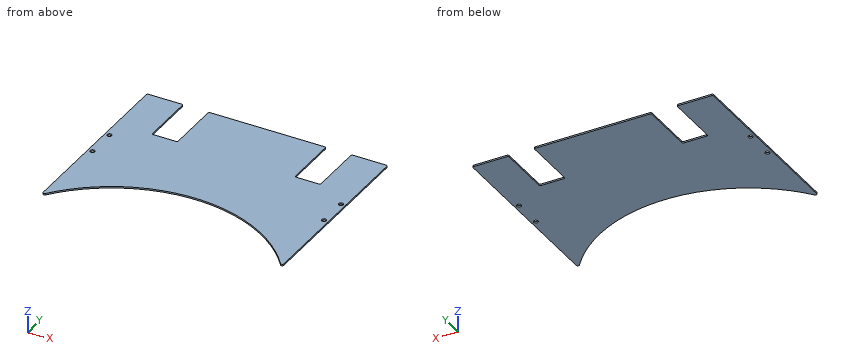
from build123d import *

# Parameters (mm, degrees)
SKETCH_1_W           = 160
SKETCH_1_H           = 104
EXTRUDE_1_DEPTH      = 0.5
SKETCH_12_R          = 99.362749495
CUT_EXTRUDE_6_DEPTH  = 1
EXTRUDE_3_DEPTH      = 1
SKETCH_17_W          = 17
SKETCH_17_H          = 92.283863988
CUT_EXTRUDE_9_DEPTH  = 1
SKETCH_21_R          = 1.525
CUT_EXTRUDE_14_DEPTH = 10
FILLET_4_R           = 1


with BuildPart() as part:
    # 草图1 → 凸台-拉伸1 (new, symmetric)
    with BuildSketch(Plane.XY):
        Rectangle(SKETCH_1_W, SKETCH_1_H)
    extrude(amount=EXTRUDE_1_DEPTH, both=True)

    # 草图12 → 切除-拉伸6 (cut)
    with BuildSketch(Plane(origin=(0, 0, -0.5), x_dir=(-1, 0, 0), z_dir=(0, 0, -1))):
        with Locations((0, -133)):
            Circle(SKETCH_12_R)
    extrude(amount=-CUT_EXTRUDE_6_DEPTH, mode=Mode.SUBTRACT)

    # 草图13 → 凸台-拉伸3 (add)
    with BuildSketch(Plane(origin=(0, 0, -0.5), x_dir=(-1, 0, 0), z_dir=(0, 0, -1))):
        with BuildLine():
            Line((80, -52), (80, -74.068209027))
            ThreePointArc((80, -74.068209027), (69.654320002, -62.139350184), (57.549595892, -52))
            Line((57.549595892, -52), (80, -52))
        make_face()
    extrude_3 = extrude(amount=-EXTRUDE_3_DEPTH)

    # 镜向2: 凸台-拉伸3 across plane
    add(extrude_3.mirror(Plane(origin=(0, 0, 0), x_dir=(0, 0, 1), z_dir=(1, 0, 0))))

    # 草图17 → 切除-拉伸9 (cut)
    with BuildSketch(Plane(origin=(0, 0, -0.5), x_dir=(-1, 0, 0), z_dir=(0, 0, -1))):
        with Locations((-47.5, 61.084572681)):
            Rectangle(SKETCH_17_W, SKETCH_17_H)
    cut_extrude_9 = extrude(amount=-CUT_EXTRUDE_9_DEPTH, mode=Mode.SUBTRACT)

    # 镜向4: 切除-拉伸9 across plane
    add(cut_extrude_9.mirror(Plane(origin=(0, 0, 0), x_dir=(0, 0, 1), z_dir=(1, 0, 0))), mode=Mode.SUBTRACT)

    # 草图21 → 切除-拉伸14 (cut)
    with BuildSketch(Plane(origin=(0, 0, -0.5), x_dir=(-1, 0, 0), z_dir=(0, 0, -1))):
        with Locations((-77, 2)):
            Circle(SKETCH_21_R)
        with Locations((-77, -18)):
            Circle(SKETCH_21_R)
        with Locations((77, -18)):
            Circle(SKETCH_21_R)
        with Locations((77, 2)):
            Circle(SKETCH_21_R)
    extrude(amount=-CUT_EXTRUDE_14_DEPTH, mode=Mode.SUBTRACT)

    # 圆角4
    fillet_4_edges = [part.edges().sort_by_distance(p)[0] for p in [
        (-80, -74.068209027, 0),
        (80, -74.068209027, 0),
        (39, 52, 0),
        (56, 52, 0),
        (56, 14.942640687, 0),
        (39, 14.942640687, 0),
        (-39, 14.942640687, 0),
        (-56, 14.942640687, 0),
        (-56, 52, 0),
        (-39, 52, 0),
        (-80, 52, 0),
        (80, 52, 0),
    ]]
    fillet(fillet_4_edges, radius=FILLET_4_R)


solid = part.part
Geometry: final body of the model. Coordinates: model frame, mm. Give positions to 0.01 mm unless a question says otherwise; leave off trailing zeros. Order: outer loops, then holes, each group sorted by start corner. A loop starts at its lowest first (then second) coordinate and runs counter-clockwise, first axis right, second up. Notation, with made-up numbers: (15, 29) -> (46, 29) arc R12 cw to (46, 44) -> close; hole circle Ø1 at (10, 5). An arc over 180 degrees is marked (long way). Answer as a JSON object with one key per item and string values.
Q1. Material intervals for probe 1 along X at (y, z) = (19, -0.05); probe 2 along Y at (x, z) = (-77, -0.2) (3 decimals); probe 3 along X at (y, z) = (-65, 0.45), sorted ascending.
Entries:
{"probe 1": "x = -80 to -56, -39 to 39, 56 to 80", "probe 2": "y = -70.199 to -19.525, -16.475 to 0.475, 3.525 to 52", "probe 3": "x = -80 to -72.45, 72.45 to 80"}
Q2. Section C-C (x = -63). Output: boundary loops of the cut face in (y, z).
Entries:
{"outline": "(-56.16, -0.5) -> (52, -0.5) -> (52, 0.5) -> (-56.16, 0.5) -> close"}
Q3. Section B-B (z = -0.35). State how many separate pieces and enclosed holes the cut face has, plus the area to 3 significant figures.
Entries:
{"separate pieces": "1", "enclosed holes": "4", "area": "14,400 mm^2"}
Q4. Section A-A (y = 44). Output: boundary loops of the cut face in (x, z), plus the area to 3 significant figures.
Entries:
{"outline": "(-80, -0.5) -> (-56, -0.5) -> (-56, 0.5) -> (-80, 0.5) -> close; (-39, -0.5) -> (39, -0.5) -> (39, 0.5) -> (-39, 0.5) -> close; (56, -0.5) -> (80, -0.5) -> (80, 0.5) -> (56, 0.5) -> close", "area": "126 mm^2"}
Q5. First-contact query: pin 1 (3.5 mm diameter, centred on x = 77, y = 2, fed in from +Z); pin 2 (3 mm diameter, centred on x = -54, y = 17.5, fed in from +Z). Flat tips, straight axial feed; report the tip coordinate or a pass-through.
Entries:
{"pin 1": "stops at z = 0.5", "pin 2": "passes through"}
